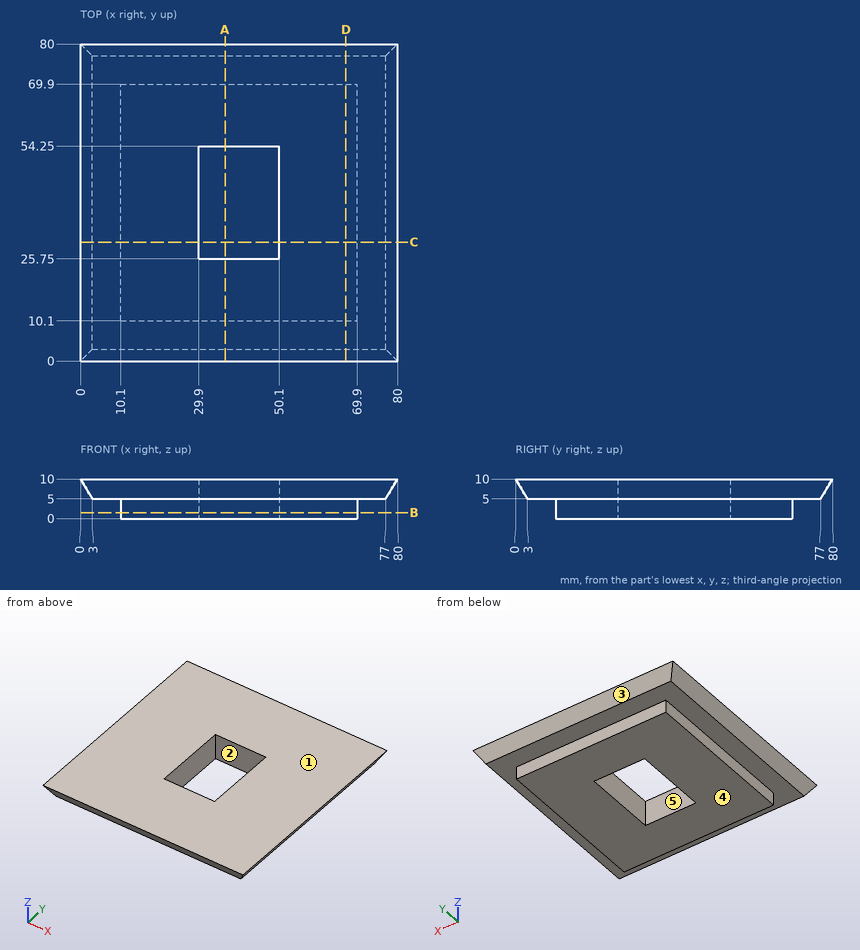
Answer from the drawing. Dimensions are ordinates in mm from the lowest x, y and z of the part. A direction names the side the tool comes from. Give positions to 0.01 mm unless a question says otherwise; leave off trailing zeros. Loops run counter-clockwise (first coordinate to the right, second up) from the corner with the lowest first, then second, coordinate; pieces in that order, holes last.
Item 1: The part is cut by section D-D (x = 67). Write down the section's boundary in (y, z), and give its area (3 significant figures).
Item 2: For the marked faces 1 and 2, determine the directions among +Z, -Z, +X, -X, +Y, -Y from which every point of the face is accessible in a straight line to the end or side of a thin tool.
Item 3: The part is cut by section B-B (z = 1.5). Write down the section's boundary in (x, y).
Item 4: The part is cut by section C-C (y = 30). Write down the section's boundary in (x, z), and give its area (3 significant figures).
Item 5: The part is cut by section A-A (x = 36.5). Write down the section's boundary in (y, z).
Item 6: The mould has two halves that part along Y. Classify the marked faces 3, 4 and 5: released by +Y, released by -Y, zero draft, split by the parting line, or undercut.
Item 7: Each of these flat-tipped pins is pushed along its axis until it touches: pin 1 Ø1.5 at (y, z) = (32.5, 1.5) entering from +X; pin 2 Ø1 at (y, z) = (15, 2.5) entering from -X; pin 3 Ø2.5 at (x, z) = (54.5, 2.5) entering from +Y; pin 4 Ø4 at (x, y) = (19, 23.5) entering from -Z. Where does it stop, or does it pass through?
Item 8: Find the intervals of material crossed by line 1 along Y through (x, z) = (41, 1); line 2 along X through (y, z) = (38, 1.75); line 3 along Z through (x, y) = (74.5, 43), in increasing order.
Taken from the geometry:
1. outline: (0, 10) - (3, 5) - (10.1, 5) - (10.1, 0) - (69.9, 0) - (69.9, 5) - (77, 5) - (80, 10) - close
1. area: 684 mm2
2. face 1: +Z, +X, -X, +Y, -Y
2. face 2: +Z, -Z
3. outline: (10.1, 10.1) - (69.9, 10.1) - (69.9, 69.9) - (10.1, 69.9) - close; hole (29.9, 25.75) - (50.1, 25.75) - (50.1, 54.25) - (29.9, 54.25) - close
4. outline: (0, 10) - (3, 5) - (10.1, 5) - (10.1, 0) - (29.9, 0) - (29.9, 10) - close; (50.1, 0) - (69.9, 0) - (69.9, 5) - (77, 5) - (80, 10) - (50.1, 10) - close
4. area: 482 mm2
5. outline: (0, 10) - (3, 5) - (10.1, 5) - (10.1, 0) - (25.75, 0) - (25.75, 10) - close; (54.25, 0) - (69.9, 0) - (69.9, 5) - (77, 5) - (80, 10) - (54.25, 10) - close
6. face 3: released by +Y
6. face 4: zero draft
6. face 5: undercut
7. pin 1: stops at x = 69.9
7. pin 2: stops at x = 10.1
7. pin 3: stops at y = 69.9
7. pin 4: stops at z = 0
8. line 1: y = 10.1 to 25.75, 54.25 to 69.9
8. line 2: x = 10.1 to 29.9, 50.1 to 69.9
8. line 3: z = 5 to 10
